Design review of the part built by this model. Coordinates are the model's own, in mm. A direction names the side the tool comes from. Coordinates: 2 decimals unless noted, no trailing zeros. Order: outer loops, then holes, each group sorted by start corner. A loop starts at its lowest first (then second) coordinate and runs counter-clockwise, first axis right, second up. Notation, with made-up numbers: (71.25, 84.5) -> (77.25, 84.5) arc R9 cw to (77.25, 96.5) -> close; hole circle Ø8 at (-35.5, 23.5). An arc over 180 degrees is marked (long way). Write item = value, one per line.
```python
from build123d import *

# Parameters (mm, degrees)
BOSS_EXTRUDE2_DEPTH = 14.3256
SKETCH3_W           = 9.2456
SKETCH3_H           = 41.8592
CUT_EXTRUDE1_DEPTH  = 14.3256
SKETCH5_W           = 2.54
SKETCH5_H           = 25.4
CUT_EXTRUDE2_DEPTH  = 14.3256
SKETCH6_R           = 1.8923
SKETCH6_R_2         = 4.1656
CUT_EXTRUDE3_DEPTH  = 14.3256


with BuildPart() as part:
    # Sketch1 → Boss-Extrude2 (new body)
    with BuildSketch(Plane.XY):
        Polygon((-1.591692429, -17.789476976), (12.708507571, -17.789476976), (12.708507571, 24.069723024), (-6.692780338, 60.558238657), (-10.104996335, 59.08528636), (-3.971611665, 44.635937574), (-12.575754632, 40.98369557), (-1.591692429, 24.069723024), align=None)
    extrude(amount=BOSS_EXTRUDE2_DEPTH)

    # Sketch3 → Cut-Extrude1 (cut)
    with BuildSketch(Plane(origin=(12.708507571, 0, 0), x_dir=(0, 0, -1), z_dir=(1, 0, 0))):
        with Locations((-7.1628, 3.140123024)):
            Rectangle(SKETCH3_W, SKETCH3_H)
    extrude(amount=-CUT_EXTRUDE1_DEPTH, mode=Mode.SUBTRACT)

    # Sketch5 → Cut-Extrude2 (cut)
    with BuildSketch(Plane(origin=(12.708507571, 0, 0), x_dir=(0, 0, -1), z_dir=(1, 0, 0))):
        with Locations((-1.27, -5.089476976)):
            Rectangle(SKETCH5_W, SKETCH5_H)
    extrude(amount=-CUT_EXTRUDE2_DEPTH, mode=Mode.SUBTRACT)

    # Sketch6 → Cut-Extrude3 (cut)
    with BuildSketch(Plane.XY.offset(14.3256)):
        with Locations((5.558407571, -13.522276976)):
            Circle(SKETCH6_R)
        with Locations((5.558407571, 10.760123024)):
            Circle(SKETCH6_R)
        with Locations((5.558407571, -2.016076976)):
            Circle(SKETCH6_R_2)
    extrude(amount=-CUT_EXTRUDE3_DEPTH, mode=Mode.SUBTRACT)


solid = part.part
```
(1) For L1, parallel to Z at x = 0.25, y = 20; L2, parallel to Y at x = -8.5, z = 13.5; L3, parallel to X at y = -4, z = 12.5, list the stretches that pass through material, from the lowest coordinate up.
Report:
L1 = 0 to 2.54, 11.79 to 14.33
L2 = 34.71 to 42.71, 55.3 to 59.78
L3 = -1.59 to 1.9, 9.22 to 12.71
(2) The part is to be moulded in two halves that separate along Z. For faces 4 (the flat face through (6, 3, 11.786)), 5 (the flat face through (3, 22, 14.326)), 6 (the flat face through (6, 24.07, 7)), 7 (the cylindrical face through (7.363, 11.329, 13.073)), say which applies: released by +Z, released by -Z, zero draft, split by the parting line, or undercut.
Report:
face_4 = undercut
face_5 = released by +Z
face_6 = undercut
face_7 = zero draft
(3) We need section D-D (y = 10). Write out the cut boundary in (x, z).
Report:
outline = (-1.59, 0) -> (3.83, 0) -> (3.83, 2.54) -> (-1.59, 2.54) -> close; (-1.59, 11.79) -> (3.83, 11.79) -> (3.83, 14.33) -> (-1.59, 14.33) -> close; (7.29, 0) -> (12.71, 0) -> (12.71, 2.54) -> (7.29, 2.54) -> close; (7.29, 11.79) -> (12.71, 11.79) -> (12.71, 14.33) -> (7.29, 14.33) -> close
(4) We need section B-B (x = -5.5). Write out the cut boundary in (y, z), and give its area (3 significant figures).
Report:
outline = (30.09, 0) -> (43.99, 0) -> (43.99, 14.33) -> (30.09, 14.33) -> close; (48.24, 0) -> (58.31, 0) -> (58.31, 14.33) -> (48.24, 14.33) -> close
area = 343 mm²
(5) For faces 1 (the flat face through (-8.213, 42.835, 7.063)), 2 (the flat face through (-1.592, 3, 13)), 3 (the flat face through (-8.38, 59.83, 7.06)), list the 3-axis set-ups (+Z, -Z, +X, -X, +Y, -Y) from which the entire face can be reached by the end or side of a thin tool; tool diameter is ignored.
Report:
face_1 = +Z, -Z, -X
face_2 = +Z, -Z, -X, -Y
face_3 = +Z, -Z, -X, +Y
(6) Insertion check: pin 1 (4.5 mm diameter, centred on x = 7.5, z = 5.5, fed in from -Y); pin 2 (4 mm diameter, centred on y = 50, z = 6.5, fed in from +X); pin 3 (3 mm diameter, centred on x = 5.56, y = -13.52, fed in from -Z); pin 4 (3 mm diameter, centred on x = -7.5, z = 11, fed in from -Y). Each pin has a flat end and moves straight along its axis. Give the tip position at first contact, or say it passes through.
Report:
pin_1 = 24.07
pin_2 = -0.02
pin_3 = through
pin_4 = 30.86
(7) We need section A-A (y = 18.5). Write out the cut boundary in (x, z).
Report:
outline = (-1.59, 0) -> (12.71, 0) -> (12.71, 2.54) -> (-1.59, 2.54) -> close; (-1.59, 11.79) -> (12.71, 11.79) -> (12.71, 14.33) -> (-1.59, 14.33) -> close
(8) We need section C-C (z = 12.75). Write out the cut boundary in (x, y) (1 decimal).
Report:
outline = (-12.6, 41) -> (-1.6, 24.1) -> (-1.6, -17.8) -> (12.7, -17.8) -> (12.7, 24.1) -> (-6.7, 60.6) -> (-10.1, 59.1) -> (-4, 44.6) -> close; hole circle Ø8.3 at (5.6, -2); hole circle Ø3.8 at (5.6, -13.5); hole circle Ø3.8 at (5.6, 10.8)
